from build123d import *

# Parameters (mm, degrees)
SKETCH2_W            = 50
SKETCH2_H            = 65
SKETCH2_R            = 2
SKETCH2_R_2          = 4
BOSS_EXTRUDE1_DEPTH  = 5
SKETCH3_W            = 21
SKETCH3_H            = 65
BOSS_EXTRUDE2_DEPTH  = 5
SKETCH4_W            = 1
SKETCH4_H            = 65
BOSS_EXTRUDE3_DEPTH  = 5
BOSS_EXTRUDE4_DEPTH  = 5
SKETCH6_R            = 2
CUT_EXTRUDE1_DEPTH   = 59
SKETCH7_R            = 1.5
CUT_EXTRUDE2_DEPTH   = 10
SKETCH7_4_R          = 1.5
CUT_EXTRUDE3_DEPTH   = 10
SKETCH7_5_R          = 1.5
BOSS_EXTRUDE5_DEPTH  = 5
SKETCH8_R            = 2
CUT_EXTRUDE4_DEPTH   = 10
SKETCH9_R            = 2.5
CUT_EXTRUDE5_DEPTH   = 10
SKETCH10_R           = 2.5
BOSS_EXTRUDE6_DEPTH  = 5
SKETCH10_4_R         = 2.5
CUT_EXTRUDE6_DEPTH   = 10
SKETCH11_W           = 72
SKETCH11_H           = 5
BOSS_EXTRUDE7_DEPTH  = 10
SKETCH12_W           = 5
SKETCH12_H           = 17.5
BOSS_EXTRUDE8_DEPTH  = 10
SKETCH14_W           = 5
SKETCH14_H           = 27.5
BOSS_EXTRUDE9_DEPTH  = 10
SKETCH13_W           = 5
SKETCH13_H           = 30
BOSS_EXTRUDE10_DEPTH = 10
SKETCH17_R           = 2
BOSS_EXTRUDE11_DEPTH = 5
SKETCH17_3_R         = 2
CUT_EXTRUDE7_DEPTH   = 10
SKETCH18_W           = 82
SKETCH18_H           = 5
CUT_EXTRUDE8_DEPTH   = 10
SKETCH19_R           = 2.5
BOSS_EXTRUDE12_DEPTH = 5
CUT_EXTRUDE9_DEPTH   = 10


with BuildPart() as part:
    # Sketch2 → Boss-Extrude1 (new body)
    with BuildSketch(Plane.XY):
        with Locations((25, 32.5)):
            Rectangle(SKETCH2_W, SKETCH2_H)
        with Locations((25, 59.5)):
            Circle(SKETCH2_R, mode=Mode.SUBTRACT)
        with Locations((13, 47.5)):
            Circle(SKETCH2_R, mode=Mode.SUBTRACT)
        with Locations((37, 47.5)):
            Circle(SKETCH2_R, mode=Mode.SUBTRACT)
        with Locations((25, 17.5)):
            Circle(SKETCH2_R_2, mode=Mode.SUBTRACT)
    extrude(amount=BOSS_EXTRUDE1_DEPTH)

    # Sketch3 → Boss-Extrude2 (add)
    with BuildSketch(Plane.XY.offset(5)):
        with Locations((-10.5, 32.5)):
            Rectangle(SKETCH3_W, SKETCH3_H)
    extrude(amount=-BOSS_EXTRUDE2_DEPTH)

    # Sketch4 → Boss-Extrude3 (add)
    with BuildSketch(Plane.XY.offset(5)):
        with Locations((-21.5, 32.5)):
            Rectangle(SKETCH4_W, SKETCH4_H)
    extrude(amount=-BOSS_EXTRUDE3_DEPTH)

    # Sketch5 → Boss-Extrude4 (add)
    with BuildSketch(Plane.XY.offset(5)):
        Polygon((-22, 17.5), (-22, 32.5), (-22, 47.5), (-28, 47.5), (-28, 17.5), align=None)
        Polygon((56, 17.5), (56, 47.5), (50, 47.5), (50, 32.5), (50, 17.5), align=None)
    extrude(amount=-BOSS_EXTRUDE4_DEPTH)

    # Sketch6 → Cut-Extrude1 (cut)
    with BuildSketch(Plane.XY.offset(5)):
        with Locations((25, 35.5)):
            Circle(SKETCH6_R)
    extrude(amount=-CUT_EXTRUDE1_DEPTH, mode=Mode.SUBTRACT)

    # Sketch7 → Cut-Extrude2 (cut)
    with BuildSketch(Plane.XY.offset(5)):
        with Locations((-17, 56.25)):
            Circle(SKETCH7_R)
        with Locations((45, 56.25)):
            Circle(SKETCH7_R)
    extrude(amount=-CUT_EXTRUDE2_DEPTH, mode=Mode.SUBTRACT)

    # Sketch7<4> → Cut-Extrude3 (cut)
    with BuildSketch(Plane.XY.offset(5)):
        with Locations((45, 8.75)):
            Circle(SKETCH7_4_R)
        with Locations((-17, 8.75)):
            Circle(SKETCH7_4_R)
    extrude(amount=-CUT_EXTRUDE3_DEPTH, mode=Mode.SUBTRACT)

    # Sketch7<5> → Boss-Extrude5 (add)
    with BuildSketch(Plane.XY.offset(5)):
        with Locations((-17, 56.25)):
            Circle(SKETCH7_5_R)
        with Locations((45, 56.25)):
            Circle(SKETCH7_5_R)
    extrude(amount=-BOSS_EXTRUDE5_DEPTH)

    # Sketch8 → Cut-Extrude4 (cut)
    with BuildSketch(Plane.XY.offset(5)):
        with Locations((-17, 8.75)):
            Circle(SKETCH8_R)
        with Locations((45, 8.75)):
            Circle(SKETCH8_R)
    extrude(amount=-CUT_EXTRUDE4_DEPTH, mode=Mode.SUBTRACT)

    # Sketch9 → Cut-Extrude5 (cut)
    with BuildSketch(Plane.XY.offset(5)):
        with Locations((25, 59.5)):
            Circle(SKETCH9_R)
        with Locations((25, 35.5)):
            Circle(SKETCH9_R)
        with Locations((13, 47.5)):
            Circle(SKETCH9_R)
        with Locations((37, 47.5)):
            Circle(SKETCH9_R)
    extrude(amount=-CUT_EXTRUDE5_DEPTH, mode=Mode.SUBTRACT)

    # Sketch10 → Boss-Extrude6 (add)
    with BuildSketch(Plane.XY.offset(5)):
        with BuildLine():
            Line((10.5, 47.5), (13, 47.5))
            Line((13, 47.5), (15.5, 47.5))
            ThreePointArc((15.5, 47.5), (13, 50), (10.5, 47.5))
        make_face()
        with BuildLine():
            Line((15.5, 47.5), (13, 47.5))
            Line((13, 47.5), (10.5, 47.5))
            ThreePointArc((10.5, 47.5), (13, 45), (15.5, 47.5))
        make_face()
        with Locations((25, 59.5)):
            Circle(SKETCH10_R)
        with BuildLine():
            ThreePointArc((39.5, 47.5), (37, 50), (34.5, 47.5))
            Line((34.5, 47.5), (37, 47.5))
            Line((37, 47.5), (39.5, 47.5))
        make_face()
        with BuildLine():
            Line((37, 47.5), (34.5, 47.5))
            ThreePointArc((34.5, 47.5), (37, 45), (39.5, 47.5))
            Line((39.5, 47.5), (37, 47.5))
        make_face()
        with Locations((25, 35.5)):
            Circle(SKETCH10_R)
    extrude(amount=-BOSS_EXTRUDE6_DEPTH)

    # Sketch10<4> → Cut-Extrude6 (cut)
    with BuildSketch(Plane.XY.offset(5)):
        with Locations((6.5, 47.5)):
            Circle(SKETCH10_4_R)
        with Locations((43.5, 47.5)):
            Circle(SKETCH10_4_R)
    extrude(amount=-CUT_EXTRUDE6_DEPTH, mode=Mode.SUBTRACT)

    # Sketch11 → Boss-Extrude7 (add)
    with BuildSketch(Plane(origin=(0, 65, 0), x_dir=(1, 0, 0), z_dir=(0, 1, 0))):
        with Locations((14, -2.5)):
            Rectangle(SKETCH11_W, SKETCH11_H)
    extrude(amount=BOSS_EXTRUDE7_DEPTH)

    # Sketch12 → Boss-Extrude8 (add)
    with BuildSketch(Plane(origin=(50, 0, 0), x_dir=(0, 0, -1), z_dir=(1, 0, 0))):
        with Locations((-2.5, 8.75)):
            Rectangle(SKETCH12_W, SKETCH12_H)
    extrude(amount=BOSS_EXTRUDE8_DEPTH)

    # Sketch14 → Boss-Extrude9 (add)
    with BuildSketch(Plane(origin=(50, 0, 0), x_dir=(0, 0, -1), z_dir=(1, 0, 0))):
        with Locations((-2.5, 61.25)):
            Rectangle(SKETCH14_W, SKETCH14_H)
    extrude(amount=BOSS_EXTRUDE9_DEPTH)

    # Sketch13 → Boss-Extrude10 (add)
    with BuildSketch(Plane(origin=(56, 0, 0), x_dir=(0, 0, -1), z_dir=(1, 0, 0))):
        with Locations((-2.5, 32.5)):
            Rectangle(SKETCH13_W, SKETCH13_H)
    extrude(amount=BOSS_EXTRUDE10_DEPTH)

    # Sketch17 → Boss-Extrude11 (add)
    with BuildSketch(Plane.XY.offset(5)):
        with Locations((45, 8.75)):
            Circle(SKETCH17_R)
        with Locations((55, 8.75)):
            Circle(SKETCH17_R)
    extrude(amount=-BOSS_EXTRUDE11_DEPTH)

    # Sketch17<3> → Cut-Extrude7 (cut)
    with BuildSketch(Plane.XY.offset(5)):
        with Locations((55, 8.75)):
            Circle(SKETCH17_3_R)
    extrude(amount=-CUT_EXTRUDE7_DEPTH, mode=Mode.SUBTRACT)

    # Sketch18 → Cut-Extrude8 (cut)
    with BuildSketch(Plane(origin=(0, 75, 0), x_dir=(1, 0, 0), z_dir=(0, 1, 0))):
        with Locations((19, -2.5)):
            Rectangle(SKETCH18_W, SKETCH18_H)
    extrude(amount=-CUT_EXTRUDE8_DEPTH, mode=Mode.SUBTRACT)

    # Sketch19 → Boss-Extrude12 (add)
    with BuildSketch(Plane.XY.offset(5)):
        with Locations((6.5, 47.5)):
            Circle(SKETCH19_R)
        with Locations((13, 47.5)):
            Circle(SKETCH19_R)
        with Locations((37, 47.5)):
            Circle(SKETCH19_R)
        with Locations((43.5, 47.5)):
            Circle(SKETCH19_R)
    extrude(amount=-BOSS_EXTRUDE12_DEPTH)

    # Sketch19<3> → Cut-Extrude9 (cut)
    with BuildSketch(Plane.XY.offset(5)):
        with BuildLine():
            Line((10.5, 47.5), (13, 47.5))
            Line((13, 47.5), (15.5, 47.5))
            ThreePointArc((15.5, 47.5), (13, 50), (10.5, 47.5))
        make_face()
        with BuildLine():
            Line((15.5, 47.5), (13, 47.5))
            Line((13, 47.5), (10.5, 47.5))
            ThreePointArc((10.5, 47.5), (13, 45), (15.5, 47.5))
        make_face()
        with BuildLine():
            ThreePointArc((39.5, 47.5), (37, 50), (34.5, 47.5))
            Line((34.5, 47.5), (37, 47.5))
            Line((37, 47.5), (39.5, 47.5))
        make_face()
        with BuildLine():
            Line((37, 47.5), (34.5, 47.5))
            ThreePointArc((34.5, 47.5), (37, 45), (39.5, 47.5))
            Line((39.5, 47.5), (37, 47.5))
        make_face()
    extrude(amount=-CUT_EXTRUDE9_DEPTH, mode=Mode.SUBTRACT)


solid = part.part
Source: CAD feature listing. Evaluate the final solid. Frame: model axes, mm. A direction names the side the tool comes from. Coordinates: 2 decimals unless noted, no trailing zeros. Loops run counter-clockwise (first coordinate to the right, second up) from the corner with the lowest first, then second, coordinate; pieces in that order, holes last. Notation, with made-up numbers: (-31.75, 24) -> (-15.75, 24) arc R20 ccw to (-15.75, 58) -> close; hole circle Ø4 at (60.25, 44). An arc over 180 degrees is marked (long way). Answer in a Markdown table with one row per item. Add a question column.
Q1. Pull-direction query (Y, two-part tool) for faces 1 (the face through (53.526, 10.102, 2.535)), 2 (the face through (18, 0, 3)), 3 (the face through (18, 32, 0)); classes: pulls with the +Y half, pulls with the -Y half, needs draft (parallel to the pull), parting line crosses it, or undercut.
Q2. Section D-D on y = 16.5. Return the cut outline in (x, z).
Q3. Reachability of faces 4 (the face through (-25, 47.5, 3)), 5 (the face through (-25, 17.5, 3)), 6 (the face through (60, 9, 3)), 7 (the face through (34.69, 48.46, 2.54)), 8 (the face through (60, 56, 3)) from +Z, -Z, +X, -X, +Y, -Y: full face, straight path, thin tool, end or side. Return the list, or none.
Q4. Contact query for flat-ended pins moving along their axis: pin 1 Ø4 at (x, y) = (-10.5, 57) entering from -Z; pin 2 Ø2 at (y, z) = (16, 1.5) entering from -X. Output: stop coordinate, or through.
Q5. Section A-A on x = 37. Return the cut outline in (y, z).
Q6. Section C-C on y = 8.75. Return the cut outline in (x, z).
Q7. Section B-B on z = 3.4. Return the cut outline in (x, y), and give its area (3 significant figures).
Q8. Ray query, line 1 along Y through (x, z) = (55, 2.6); line 2 along Y through (x, z) = (25, 1.1); line 3 along X through (y, z) = (52, 4.4). Return the intervals inside material, ascending.
Computed values:
| question | item | result |
|---|---|---|
| 1 | face 1 | undercut |
| 1 | face 2 | pulls with the -Y half |
| 1 | face 3 | needs draft |
| 2 | outline | (-22, 0) -> (21.13, 0) -> (21.13, 5) -> (-22, 5) -> close; (28.87, 0) -> (60, 0) -> (60, 5) -> (28.87, 5) -> close |
| 3 | face 4 | +Z, -Z, -X, +Y |
| 3 | face 5 | +Z, -Z, -X, -Y |
| 3 | face 6 | +Z, -Z, +X, -Y |
| 3 | face 7 | +Z, -Z |
| 3 | face 8 | +Z, -Z, +X, +Y |
| 4 | pin 1 | stops at z = 0 |
| 4 | pin 2 | stops at x = -22 |
| 5 | outline | (0, 0) -> (45, 0) -> (45, 5) -> (0, 5) -> close; (50, 0) -> (65, 0) -> (65, 5) -> (50, 5) -> close |
| 6 | outline | (-22, 0) -> (-19, 0) -> (-19, 5) -> (-22, 5) -> close; (-15, 0) -> (53, 0) -> (53, 5) -> (-15, 5) -> close; (57, 0) -> (60, 0) -> (60, 5) -> (57, 5) -> close |
| 7 | outline | (-28, 17.5) -> (-22, 17.5) -> (-22, 0) -> (60, 0) -> (60, 17.5) -> (66, 17.5) -> (66, 47.5) -> (60, 47.5) -> (60, 65) -> (-22, 65) -> (-22, 47.5) -> (-28, 47.5) -> close; hole circle Ø4 at (-17, 8.75); hole circle Ø5 at (13, 47.5); hole circle Ø8 at (25, 17.5); hole circle Ø5 at (37, 47.5); hole circle Ø4 at (55, 8.75) |
| 7 | area | 5,580 mm^2 |
| 8 | line 1 | y = 0 to 6.75, 10.75 to 65 |
| 8 | line 2 | y = 0 to 13.5, 21.5 to 65 |
| 8 | line 3 | x = -22 to 60 |
